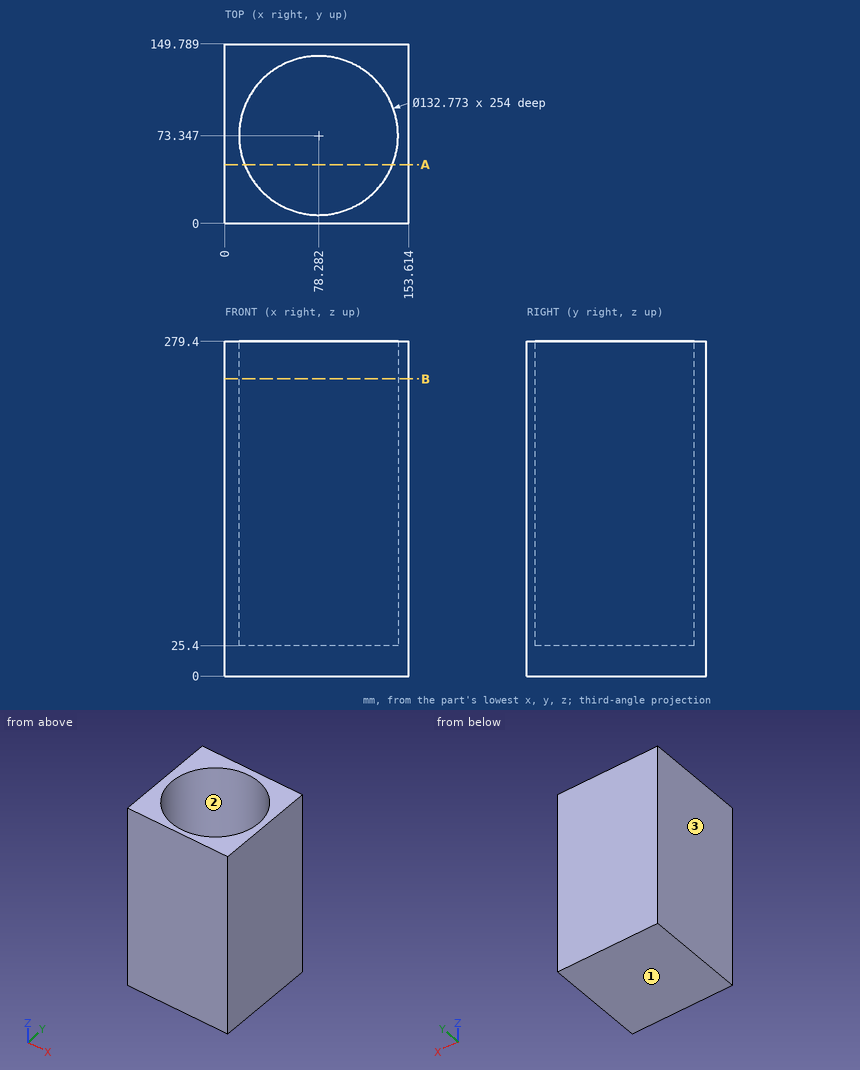
Job drawing, mm, ordinate dimensions from the low corner. One solid piece. Round coordinates to 2 decimals unless told otherwise and drop trailing zeros. Order: outer loops, then holes, each group sorted by start corner. A loop starts at its lowest first (then second) coordinate and runs counter-clockwise, first axis right, second up. Notation, with made-up numbers: M 14,-10.5 L 50,-10.5 A7 cw 50,1.5 Z; hole C -24,57.5 d11. An arc over 180 degrees is marked long. Write each question's results on one line, items separated by ' | '. Start each with the question number.
(1) Drop flat-ended pins along their axis: pin 1 (3 mm diameter, centred on y = 92.5, z = 102, fed in from -X); pin 2 (3 mm diameter, centred on x = 67.5, y = 90.5, fed in from +Z). Give the stop position or say it passes through.
(2) Saw through at B-B, the plane z = 248. Give the cut face in (x, y).
(3) Two-plate mould, pull along X, no slides. Class the marked faces 1, 2 and 3: pulls with the +X half, pulls with the -X half, needs draft (parallel to the pull), parting line crosses it, or undercut.
(4) Saw through at A-A, the plane y = 49. Give the cut face in (x, z).
(5) Probe probe 1 along Y at (x, z) = (79, 154.5) (1 decimal); probe 2 along Z at (x, y) = (63.5, 63); probe 3 along X at (y, z) = (36.5, 77.5) (1 decimal). List the from-to ranges inside material, lowest first. Write a range as from..to.
Established:
1) pin 1: stops at x = 0 | pin 2: stops at z = 25.4
2) outline: M 0,0 L 153.61,0 L 153.61,149.79 L 0,149.79 Z; hole C 78.28,73.35 d132.77
3) face 1: needs draft | face 2: undercut | face 3: pulls with the -X half
4) outline: M 0,0 L 153.61,0 L 153.61,279.4 L 140.04,279.4 L 140.04,25.4 L 16.52,25.4 L 16.52,279.4 L 0,279.4 Z
5) probe 1: y = 0..7, 139.7..149.8 | probe 2: z = 0..25.4 | probe 3: x = 0..23.1, 133.5..153.6
